Input: part model. Units: mm. Frame: model coordinates. Face numbers are marked on the shaded views. Give positions to 0.01 mm unless a question says otherwise; leave off trailing zeros. Loops run counter-clockwise (first coordinate to the right, second up) from the corner with the lowest first, then second, coordinate; pieces in that order, holes last. Notation, with made-up numbers: (-2.5, 81) -> (36.5, 81) arc R28 ccw to (36.5, 103) -> close; hole circle Ø10 at (-5, 66). An arc over 180 degrees is marked (long way). One line per question, with ' | ' between items.
from build123d import *

# Parameters (mm, degrees)
F2_ANGLE = 180


with BuildPart() as f2:
    # F1 (on Front) → F2 (revolve)
    with BuildSketch(Plane.XZ):
        Polygon((-44.861279428, 12.9604106769), (-51.217135042, 12.9604106769), (-57.5630575919, 12.9604106769), (-57.5630575919, 15.2494033683), (-58.6807462598, 15.475716571), (-60.8853201683, 14.20289014), (-61.2508664965, 13.1247800337), (-59.2498548651, 11.9714734282), (-62.425474964, 6.4711380712), (-65.6057968908, 0.9626589096), (-67.5986398816, 2.1112574229), (-68.3491751552, 1.2704479365), (-68.3491751552, -1.2704479365), (-67.590510429, -2.1238883528), (-65.6038210217, -0.9768590888), (-62.4301136979, -6.4738162454), (-59.2582268861, -11.9676853595), (-61.244893976, -13.1146881387), (-60.8774400163, -14.19364456), (-58.6706588228, -15.4396259846), (-57.5584731996, -15.2283469215), (-57.5584731996, -12.9530243576), (-51.217135042, -12.9530243576), (-44.862665236, -12.9530243576), (-44.862665236, -15.2283469215), (-43.7646710275, -15.4396259846), (-41.5434874137, -14.2077057619), (-41.1808964662, -13.1190662144), (-43.1607244284, -11.9802929242), (-39.9959231548, -6.4780897113), (-36.8304619331, -0.9747391376), (-34.850633971, -2.1135124278), (-34.0965986252, -1.2640794445), (-34.1053716838, 1.2640794445), (-34.8630113186, 2.1323707922), (-36.8285001335, 0.9983813071), (-39.9917026714, 6.4810064009), (-43.1661904902, 11.9793805911), (-41.19939244, 13.1149119748), (-41.5604028179, 14.1900196116), (-43.7584016402, 15.4673718757), (-44.861279428, 15.2523063589), align=None)
        Polygon((-60.7503676631, -13.9712226825), (-58.5499524964, -12.7008123937), (-58.5499524964, -15.2283469215), align=None, mode=Mode.SUBTRACT)
        Polygon((-68.0832503253, 1.2704479365), (-65.8827699508, 0), (-68.0832503253, -1.2704479365), align=None, mode=Mode.SUBTRACT)
        Polygon((-43.8843175875, -15.2283469215), (-43.8843175875, -12.7008123937), (-41.6742515512, -13.9767946147), align=None, mode=Mode.SUBTRACT)
        with BuildLine():
            ThreePointArc((-51.217135042, 12.7008123937), (-42.2363044718, 8.9808305702), (-38.5163226482, 0))
            ThreePointArc((-38.5163226482, 0), (-60.1979656121, -8.9808305702), (-51.217135042, 12.7008123937))
        make_face(mode=Mode.SUBTRACT)
        Polygon((-34.3620503103, -1.2640794445), (-36.5515001331, 0), (-34.3620503103, 1.2640794445), align=None, mode=Mode.SUBTRACT)
        Polygon((-58.5499524964, 15.2491778135), (-58.5499524964, 12.7008123937), (-60.7598529608, 13.9766990217), align=None, mode=Mode.SUBTRACT)
        Polygon((-41.6910577545, 13.9670915487), (-43.8843175875, 12.7008123937), (-43.8843175875, 15.2525296435), align=None, mode=Mode.SUBTRACT)
    revolve(axis=Axis((0, 0, 0), (0, 0, 1)), revolution_arc=F2_ANGLE)


solid = f2.part
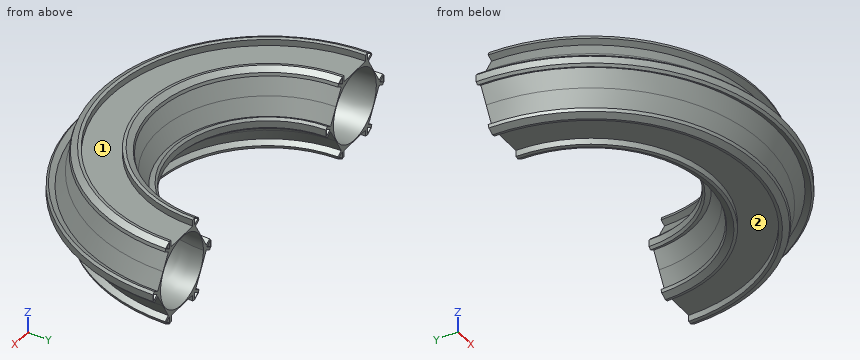
1. Section query B-B (z = 10). Output: boundary loops of the cut face in (x, y), then the cut area to 4 significant figures.
Determined:
outline: (-60.39, 0) arc R60.39 ccw to (60.39, 0) -> (59.05, 0) arc R59.05 cw to (-59.05, 0) -> close; (-43.39, 0) arc R43.39 ccw to (43.39, 0) -> (42.02, 0) arc R42.02 cw to (-42.02, 0) -> close | area: 434.5 mm2
2. Ray query, line 1 along X through (y, z) = (-4.5, -11); line 2 along Z through (x, y) = (-16, -53); line 3 along X through (y, z) = (-10, 6). Return the intervals inside material, ascending. Write a range as from..to.
Determined:
line 1: x = -59.65..-57.39, -44.64..-42.36, 42.36..44.64, 57.39..59.65 | line 2: z = -12.95..-12.01, 12.01..12.96 | line 3: x = -61.89..-61.61, -38.75..-38.43, 38.43..38.75, 61.61..61.89
3. Pin query (flat end, axial travel): P1, Ø5, axis at x = -3.5, y = -36, coming from the +Z side; P2, Ø4, axis at y = -19.5, z = -1, coming from the -X side; P3, Ø10, axis at y = -47, z = -0.5, coming from the +X side; P4, Ø17.5, axis at x = 23, y = -29.5, coming from the -Z side. Return the tip coordinate at first contact, or that it passes through.
Determined:
P1: stops at z = 4.19 | P2: stops at x = -66.07 | P3: stops at x = 53.92 | P4: stops at z = -15.44
4. Section query A-A (z = -9.5). Output: boundary loops of the cut face in (x, y).
Determined:
outline: (-60.68, 0) arc R60.68 ccw to (60.68, 0) -> (59.65, 0) arc R59.65 cw to (-59.65, 0) -> close; (-42.79, 0) arc R42.79 ccw to (42.79, 0) -> (41.73, 0) arc R41.73 cw to (-41.73, 0) -> close
5. Section query C-C (y = -16.5). Count the separate pieces of the cut face and the enclosed holes in it, then the cut area to 3 significant figures.
Determined:
separate pieces: 2 | enclosed holes: 14 | area: 227 mm2
6. Pull-direction query (X, two-part tool) for the marked faces 1 and 2; classes: pulls with the +X half, pulls with the -X half, needs draft (parallel to the pull), parting line crosses it, or undercut.
Determined:
face 1: undercut | face 2: undercut
